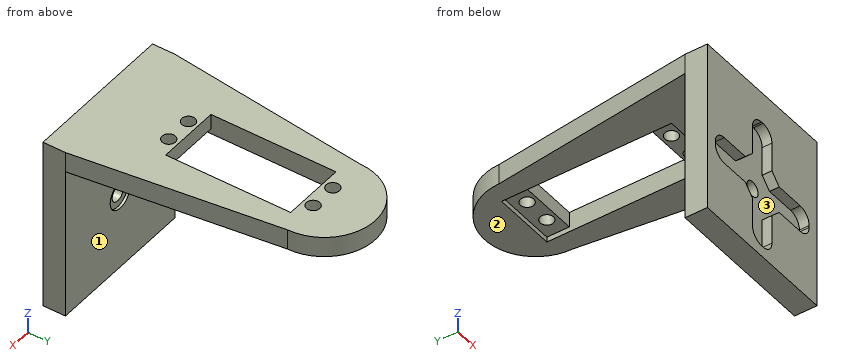
Autodesk Inventor part; units mm, degrees
ref_plane "Work Plane2" through (-15, 0, 16) normal (0, 0, 1) x (1, 0, 0)
ref_plane "YZ Plane" through (0, 0, 0) normal (1, 0, 0) x (0, 1, 0)
ref_plane "XZ Plane" through (0, 0, 0) normal (0, 1, 0) x (-1, 0, 0)
sketch "Sketch1" plane through (0, 0, 0) normal (0, 1, 0) x (-1, 0, 0)
  line L0 (-15, -15) -> (15, -15)
  line L1 (15, -15) -> (15, 15)
  line L2 (15, 15) -> (-15, 15)
  line L3 (-15, 15) -> (-15, -15)
  line L4 (-15, -15) -> (15, 15) construction
  line L5 (15, -15) -> (-15, 15) construction
  line L6 (-2.45, -12.65) -> (2.45, -12.65) construction
  line L7 (2.45, -12.65) -> (2.45, 12.65) construction
  line L8 (2.45, 12.65) -> (-2.45, 12.65) construction
  line L9 (-2.45, 12.65) -> (-2.45, -12.65) construction
  line L10 (-2.45, -12.65) -> (2.45, 12.65) construction
  line L11 (2.45, -12.65) -> (-2.45, 12.65) construction
  line L12 (-12.65, -2.45) -> (12.65, -2.45) construction
  line L13 (12.65, -2.45) -> (12.65, 2.45) construction
  line L14 (12.65, 2.45) -> (-12.65, 2.45) construction
  line L15 (-12.65, 2.45) -> (-12.65, -2.45) construction
  line L16 (-12.65, -2.45) -> (12.65, 2.45) construction
  line L17 (12.65, -2.45) -> (-12.65, 2.45) construction
  line L18 (-12.85, -2.65) -> (12.85, -2.65)
  line L19 (12.85, -2.65) -> (12.85, 2.65)
  line L20 (12.85, 2.65) -> (-12.85, 2.65)
  line L21 (-12.85, 2.65) -> (-12.85, -2.65)
  line L22 (-12.85, -2.65) -> (12.85, 2.65) construction
  line L23 (12.85, -2.65) -> (-12.85, 2.65) construction
  line L24 (-2.65, -12.85) -> (2.65, -12.85)
  line L25 (2.65, -12.85) -> (2.65, 12.85)
  line L26 (2.65, 12.85) -> (-2.65, 12.85)
  line L27 (-2.65, 12.85) -> (-2.65, -12.85)
  line L28 (-2.65, -12.85) -> (2.65, 12.85) construction
  line L29 (2.65, -12.85) -> (-2.65, 12.85) construction
  point P0 (0, 0)
  point P1 (0, 0)
  dimension "d0" = 30
  dimension "d1" = 4.9
  dimension "d2" = 10.2
  dimension "d3" = 0.2
  dimension "d4" = 0.2
extrude "Extrusion1" add sketch "Sketch1" along normal blind 1.9
sketch "Sketch2" plane through (0, 1.9, 0) normal (0, 1, 0) x (1, 0, 0)
  line L0 (15, 15) -> (-15, 15)
  line L1 (-15, 15) -> (-15, -15)
  line L2 (-15, -15) -> (15, -15)
  line L3 (15, -15) -> (15, 15)
  circle A0 centre (0, 0) radius 1.5
  dimension "d7" = 3
extrude "Extrusion2" add sketch "Sketch2" along normal blind 2
sketch "Sketch3" plane through (0, 3.9, 0) normal (0, 1, 0) x (1, 0, 0)
  circle A0 centre (0, 0) radius 1.5
  line L0 (15, 15) -> (-15, 15)
  line L1 (-15, 15) -> (-15, -15)
  line L2 (-15, -15) -> (15, -15)
  line L3 (15, -15) -> (15, 15)
  circle A1 centre (0, 0) radius 2.75
  dimension "d10" = 5.5
extrude "Extrusion3" add sketch "Sketch3" along normal blind 0.5 contours L3 L2 L1 L0
chamfer "Chamfer1" distance 2 angle 45 1 edges at (-2.65, 0.95, -2.65)
fillet "Fillet1" radius 2.45 1 edges at (-12.85, 0.95, -2.65)
fillet "Fillet2" radius 2.45 1 edges at (-2.65, 0.95, -12.85)
chamfer "Chamfer2" distance 2 angle 45 1 edges at (2.65, 0.95, -2.65)
chamfer "Chamfer3" distance 2 angle 45 1 edges at (2.65, 0.95, 2.65)
fillet "Fillet3" radius 2.45 1 edges at (12.85, 0.95, -2.65)
fillet "Fillet4" radius 2.45 1 edges at (2.65, 0.95, -12.85)
fillet "Fillet5" radius 2.45 1 edges at (12.85, 0.95, 2.65)
fillet "Fillet6" radius 2.45 1 edges at (2.65, 0.95, 12.85)
chamfer "Chamfer4" distance 2 angle 45 1 edges at (-2.65, 0.95, 2.65)
fillet "Fillet7" radius 2.45 2 edges at (-2.65, 0.95, 12.85) (-12.85, 0.95, 2.65)
sketch "Sketch8" plane through (-15, 0, 15) normal (0, 0, 1) x (1, 0, 0)
  line L0 (0, 0) -> (30, 0)
  line L1 (30, 0) -> (30, 4.4)
  line L2 (0, 4.4) -> (30, 4.4)
  line L3 (0, 0) -> (0, 4.4)
  line L4 (15, 0) -> (15, 120) construction
  line L5 (30, 4.4) -> (25, 44.4)
  line L6 (25, 44.4) -> (5, 44.4)
  line L7 (5, 44.4) -> (0, 4.4)
  arc A0 (25, 44.4) -> (5, 44.4) centre (15, 44.4) ccw
  dimension "d101" = 40
  dimension "d102" = 20
extrude "Extrusion7" add sketch "Sketch8" along normal blind 4
sketch "Sketch9" plane through (-15, 0, 19) normal (0, 0, 1) x (1, 0, 0)
  line L0 (0, 0) -> (30, 0)
  line L1 (9.3, 41.75) -> (20.7, 41.75) construction
  line L2 (20.7, 41.75) -> (20.7, 18.25) construction
  line L3 (20.7, 18.25) -> (9.3, 18.25) construction
  line L4 (9.3, 18.25) -> (9.3, 41.75) construction
  line L5 (15, 90) -> (15, 15.8225) construction
  line L6 (9.3, 41.75) -> (9.3, 46.15) construction
  line L7 (9.3, 46.15) -> (20.7, 46.15) construction
  line L8 (20.7, 46.15) -> (20.7, 41.75) construction
  line L9 (20.7, 18.25) -> (20.7, 13.85) construction
  line L10 (20.7, 13.85) -> (9.3, 13.85) construction
  line L11 (9.3, 13.85) -> (9.3, 18.25) construction
  circle A0 centre (12.3, 44.15) radius 1.3
  circle A1 centre (17.7, 44.15) radius 1.3
  line L12 (-17.4512, 30) -> (18.2205, 30) construction
  circle A2 centre (12.3, 15.85) radius 1.3
  circle A3 centre (17.7, 15.85) radius 1.3
  line L13 (8.8, 42.25) -> (21.2, 42.25)
  line L14 (21.2, 42.25) -> (21.2, 17.75)
  line L15 (21.2, 17.75) -> (8.8, 17.75)
  line L16 (8.8, 17.75) -> (8.8, 42.25)
  line L17 (15, 0) -> (15, 83.8502) construction
  dimension "d105" = 11.4
  dimension "d106" = 23.5
  dimension "d107" = 3
  dimension "d108" = 2.4
  dimension "d109" = 4.4
  dimension "d110" = 0.5
  dimension "d111" = 0.5
  dimension "d113" = 2.6
  dimension "d122" = 30
extrude "Extrusion8" cut sketch "Sketch9" against normal through all
sketch "Sketch10" plane through (-15, 0, 19) normal (0, 0, 1) x (1, 0, 0)
  circle A0 centre (17.7, 15.85) radius 1.3
  circle A1 centre (17.7, 44.15) radius 1.3
  circle A2 centre (12.3, 44.15) radius 1.3
  circle A3 centre (12.3, 15.85) radius 1.3
  line L0 (8.8, 17.75) -> (8.8, 42.25)
  line L1 (8.8, 42.25) -> (21.2, 42.25)
  line L2 (21.2, 42.25) -> (21.2, 17.75)
  line L3 (21.2, 17.75) -> (8.8, 17.75)
  line L4 (0, 0) -> (30, 0)
  line L5 (9.3, 41.75) -> (20.7, 41.75) construction
  line L6 (20.7, 41.75) -> (20.7, 18.25) construction
  line L7 (20.7, 18.25) -> (9.3, 18.25) construction
  line L8 (9.3, 18.25) -> (9.3, 41.75) construction
  line L9 (15, 87.388) -> (15, -76.2197) construction
  line L10 (9.3, 41.75) -> (9.3, 46.15) construction
  line L11 (9.3, 46.15) -> (20.7, 46.15) construction
  line L12 (20.7, 46.15) -> (20.7, 41.75) construction
  line L13 (20.7, 18.25) -> (20.7, 13.85) construction
  line L14 (20.7, 13.85) -> (9.3, 13.85) construction
  line L15 (9.3, 13.85) -> (9.3, 18.25) construction
  line L16 (0.832, 30) -> (29.7617, 30) construction
  line L17 (8.8, 46.65) -> (21.2, 46.65)
  line L18 (21.2, 46.65) -> (21.2, 13.35)
  line L19 (21.2, 13.35) -> (8.8, 13.35)
  line L20 (8.8, 13.35) -> (8.8, 46.65)
  line L21 (15, 0) -> (15, 87.4766) construction
  dimension "d125" = 11.4
  dimension "d126" = 23.5
  dimension "d127" = 4.4
  dimension "d128" = 0.5
  dimension "d130" = 0.5
  dimension "d136" = 30
ref_plane "Work Plane2" through (-15, 0, 16) normal (0, 0, 1) x (1, 0, 0)
extrude "Extrusion10" cut sketch "Sketch10" along normal up to surface (1 mm away) from surface at -4 contours L3 L18 L19 L20 | L20 L17 L18 L1
equation "\"d0\" = FrontUpperLegShoulderWidth"
equation "\"d1\" = ServoArmWidth"
equation "\"d2\" = ServoArmLength"
equation "\"d3\" = ServoArmSpacing"
equation "\"d4\" = ServoArmSpacing"
equation "\"d5\" = ServoArmThickness"
equation "\"d7\" = ServoArmHoleRequired"
equation "\"d8\" = MinimalThickness"
equation "\"d10\" = ServoArmHeadScrewTrace"
equation "\"d11\" = ServoArmHeadScrewThickness"
equation "\"d13\" = ServoArmInternFillet"
equation "\"d16\" = ServoArmExternFillet"
equation "\"d17\" = ServoArmExternFillet"
equation "\"d18\" = ServoArmInternFillet"
equation "\"d21\" = ServoArmInternFillet"
equation "\"d24\" = ServoArmExternFillet"
equation "\"d25\" = ServoArmExternFillet"
equation "\"d26\" = ServoArmExternFillet"
equation "\"d27\" = ServoArmExternFillet"
equation "\"d28\" = ServoArmInternFillet"
equation "\"d31\" = ServoArmExternFillet"
equation "\"d101\" = FrontShoulderHeight"
equation "\"d102\" = FrontShoulderWidth"
equation "\"d103\" = FrontShoulderThickness"
equation "\"d105\" = ServoCoreWidth"
equation "\"d106\" = ServoCoreLength"
equation "\"d107\" = ServoEdgeToFixation"
equation "\"d108\" = ServoCoreToFixation"
equation "\"d109\" = ServoFixationLength"
equation "\"d110\" = ServoTraceSpacing"
equation "\"d111\" = ServoTraceSpacing"
equation "\"d113\" = ServoScrewDiameterRequired"
equation "\"d122\" = FrontShoulderServoCenterDistance"
equation "\"d123\" = FrontShoulderThickness"
equation "\"d125\" = ServoCoreWidth"
equation "\"d126\" = ServoCoreLength"
equation "\"d127\" = ServoFixationLength"
equation "\"d128\" = ServoTraceSpacing"
equation "\"d130\" = ServoTraceSpacing"
equation "\"d136\" = FrontShoulderServoCenterDistance"
equation "\"ServoTraceSpacing\" = 0.5"
equation "\"FrontUpperLegShoulderWidth\" = 30"
equation "\"LegServoThickness\" = 3"
equation "\"FrontShoulderHeight\" = 40"
equation "\"FrontShoulderWidth\" = 20"
equation "\"FrontShoulderThickness\" = 4"
equation "\"FrontShoulderServoCenterDistance\" = 30"
equation "\"d140\" = -LegServoThickness"
properties part number "BackUpperLegShoulder" material "PC/ABS Plastic"
Could you check a few things on this model? Use its own coordinates, in mm. Face numbers are marked on the shaded views. Give positions to 0.01 mm unless a question says otherwise; leave off trailing zeros. Order: outer loops, then holes, each group sorted by start corner. A loop starts at its lowest first (then second) coordinate and runs counter-clockwise, first axis right, second up.
Item 1: If we section it at B-B, the plane y = 15.85: Write out the boundary of the cut face in (x, z), plus the area to 4 significant figures.
Item 2: If we section it at D-D, the plane x = -8.5: Write out the boundary of the cut face in (y, z).
Item 3: If we mould it in two halves opening along Z, with no side actions, what happens to the marked faces 1, 2 and 3? For each: pulls with the +Z half, pulls with the -Z half, needs draft (parallel to the pull), parting line crosses it, or undercut.
Item 4: If we section it at A-A, the plane y = 26: Write out the boundary of the cut face in (x, z).
Item 5: I need wall thicknesses on line 1 (X direction, y = 3.4, z = 0); line 2 (Z direction, x = 0, y = 4.1); line 3 (Y direction, x = 2, z = 17). Which ranges of each line are inside material? Lowest first, please.
Item 6: If we section it at C-C, the plane z = 9: Write out the boundary of the cut face in (x, y), plus the area to 3 significant figures.
Item 7: I'm going to push flat-ended pins straight in: pin 1 (12 mm diameter, centred on y = 9, z = 4, fed in from -X); pin 2 (4.5 mm diameter, centred on x = -1.5, z = -0.5, fed in from +Y); pin 3 (1.5 mm diameter, centred on x = -5.5, y = 13.5, fed in from -Z); pin 4 (3.5 mm diameter, centred on x = -2, y = 44, fed in from -Z). Where does each tip first touch, or does it pass through?
Values:
1. outline: (-13.57, 15) - (-6.2, 15) - (-6.2, 16) - (-4, 16) - (-4, 19) - (-13.57, 19) - close; (-1.4, 16) - (1.4, 16) - (1.4, 19) - (-1.4, 19) - close; (4, 16) - (6.2, 16) - (6.2, 15) - (13.57, 15) - (13.57, 19) - (4, 19) - close
1. area: 80.55 mm2
2. outline: (0, -15) - (4.4, -15) - (4.4, 15) - (49.67, 15) - (49.67, 19) - (0, 19) - (0, 2.65) - (1.9, 2.65) - (1.9, -2.65) - (0, -2.65) - close
3. face 1: needs draft
3. face 2: pulls with the -Z half
3. face 3: undercut
4. outline: (-12.3, 15) - (-6.2, 15) - (-6.2, 19) - (-12.3, 19) - close; (6.2, 15) - (12.3, 15) - (12.3, 19) - (6.2, 19) - close
5. line 1: x = -15 to -1.5, 1.5 to 15
5. line 2: z = -15 to -2.75, 2.75 to 19
5. line 3: y = 0 to 14.75, 16.95 to 17.75, 42.25 to 43.05, 45.25 to 54.2
6. outline: (-15, 0) - (-2.65, 0) - (-2.65, 1.9) - (2.65, 1.9) - (2.65, 0) - (15, 0) - (15, 4.4) - (-15, 4.4) - close
6. area: 122 mm2
7. pin 1: stops at x = -15
7. pin 2: stops at y = 4.4
7. pin 3: stops at z = 15
7. pin 4: stops at z = 16
